Geometry check sheet. Reference: the model listing, model coordinates, mm. Face numbers are marked on the shaded views. Give positions to 0.01 mm unless a question says otherwise; leave off trailing zeros. Order: outer loops, then holes, each group sorted by start corner. A loop starts at its lowest first (then second) coordinate and runs counter-clockwise, first axis right, second up. Notation, with made-up numbers: M 39,37 L 75,37 A11 cw 75,48 Z; hole C 74.25,35.5 d4. An arc over 180 degrees is marked long. Answer as CSV lines item,"result". Start each with the question number.
Q1. Section check D-D, the plane x = 0. Record the boundary of the cut face in (y, z).
Q2. Thickness scan on line 1 (X direction, y = 20, z = 0); line 2 (Z direction, x = 0, y = 11.5); line 3 (X direction, y = 9, z = 6.5). Record the ranges inside material, lowest first.
Q3. Section check B-B, the plane x = -7.75. Record the boundary of the cut face in (y, z) (3 decimals), then the cut area to 3 significant figures.
Q4. Section check A-A, the plane z = 0. Record the boundary of the cut face in (x, y).
Q5. Section check C-C, the plane y = 3. Record the boundary of the cut face in (x, z) (1 decimal), then the cut area to 3 significant figures.
Q6. Mould release check, pull along Z, two halves, no side actions. Record for the marked faces 1, 2, 3 and 4: +Z half, -Z half, draft (parallel to the pull), parting line (faces both ways), or undercut.
Q7. Go/stop test with flat-tipped pins: pin 1 (3 mm diameter, centred on x = 4.5, y = 13, fed in from -Z); pin 2 (6 mm diameter, centred on y = 27, z = -6, fed in from -X); pin 3 (1 mm diameter, centred on y = 16.5, z = -6, fed in from -X); pin 4 (3 mm diameter, centred on x = -4.5, z = -2.5, fed in from +Y). Record where each tip stops, or that it passes through.
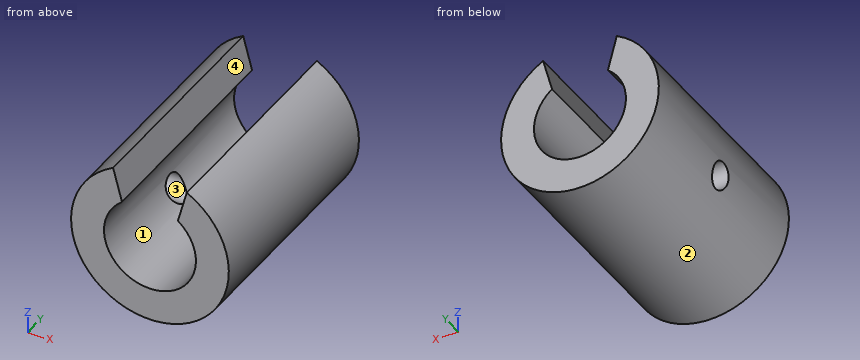
```python
from build123d import *

# Parameters (mm, degrees)
SKETCH1_R           = 11.1125
BOSS_EXTRUDE1_DEPTH = 31.75
CUT_EXTRUDE1_DEPTH  = 36.426512847
SKETCH3_R           = 1.778
CUT_EXTRUDE2_DEPTH  = 31.75


with BuildPart() as part:
    # Sketch1 → Boss-Extrude1 (new body)
    with BuildSketch(Plane(origin=(0, 0, 0), x_dir=(1, 0, 0), z_dir=(0, 1, 0))):
        with Locations(Location((0, 0, 0), (0, 0, 270))):
            Circle(SKETCH1_R)
    extrude(amount=BOSS_EXTRUDE1_DEPTH)

    # Sketch2 → Cut-Extrude1 (cut, through all)
    with BuildSketch(Plane(origin=(0, 31.75, 0), x_dir=(1, 0, 0), z_dir=(0, 1, 0))):
        with BuildLine():
            Line((-3.937, -5.14310801), (-5.191572052, -9.825234648))
            ThreePointArc((-5.191572052, -9.825234648), (0, -11.1125), (5.191572052, -9.825234648))
            Line((5.191572052, -9.825234648), (3.937, -5.14310801))
            ThreePointArc((3.937, -5.14310801), (0, 6.477), (-3.937, -5.14310801))
        make_face()
    extrude(amount=-CUT_EXTRUDE1_DEPTH, mode=Mode.SUBTRACT)

    # Sketch3 → Cut-Extrude2 (cut)
    with BuildSketch(Plane(origin=(0, 0, 0), x_dir=(0, 0, -1), z_dir=(1, 0, 0))):
        with Locations((3.175, 15.875)):
            Circle(SKETCH3_R)
    extrude(amount=-CUT_EXTRUDE2_DEPTH, mode=Mode.SUBTRACT)


solid = part.part
```
Answer block:
1,outline,"M 0,-11.11 L 31.75,-11.11 L 31.75,-6.48 L 0,-6.48 Z"
2,line 1,"x = -11.11 to -6.48, 6.48 to 11.11"
2,line 2,"z = -11.11 to -6.48"
2,line 3,"x = -9.01 to -4.3, 4.3 to 9.01"
3,outline,"M 0,-7.964 L 31.75,-7.964 L 31.75,7.964 L 0,7.964 Z; hole C 15.875,-3.175 d3.556"
3,area,"496 mm2"
4,outline,"M -11.11,0 L -6.48,0 L -6.48,31.75 L -11.11,31.75 Z; M 6.48,0 L 11.11,0 L 11.11,31.75 L 6.48,31.75 Z"
5,outline,"M -5.2,9.8 A11.1 ccw long 5.2,9.8 L 3.9,5.1 A6.5 cw long -3.9,5.1 Z"
5,area,"212 mm2"
6,face 1,"undercut"
6,face 2,"parting line"
6,face 3,"undercut"
6,face 4,"+Z half"
7,pin 1,"stops at z = -10.7"
7,pin 2,"stops at x = -10.7"
7,pin 3,"stops at x = -9.66"
7,pin 4,"stops at y = 31.75"
